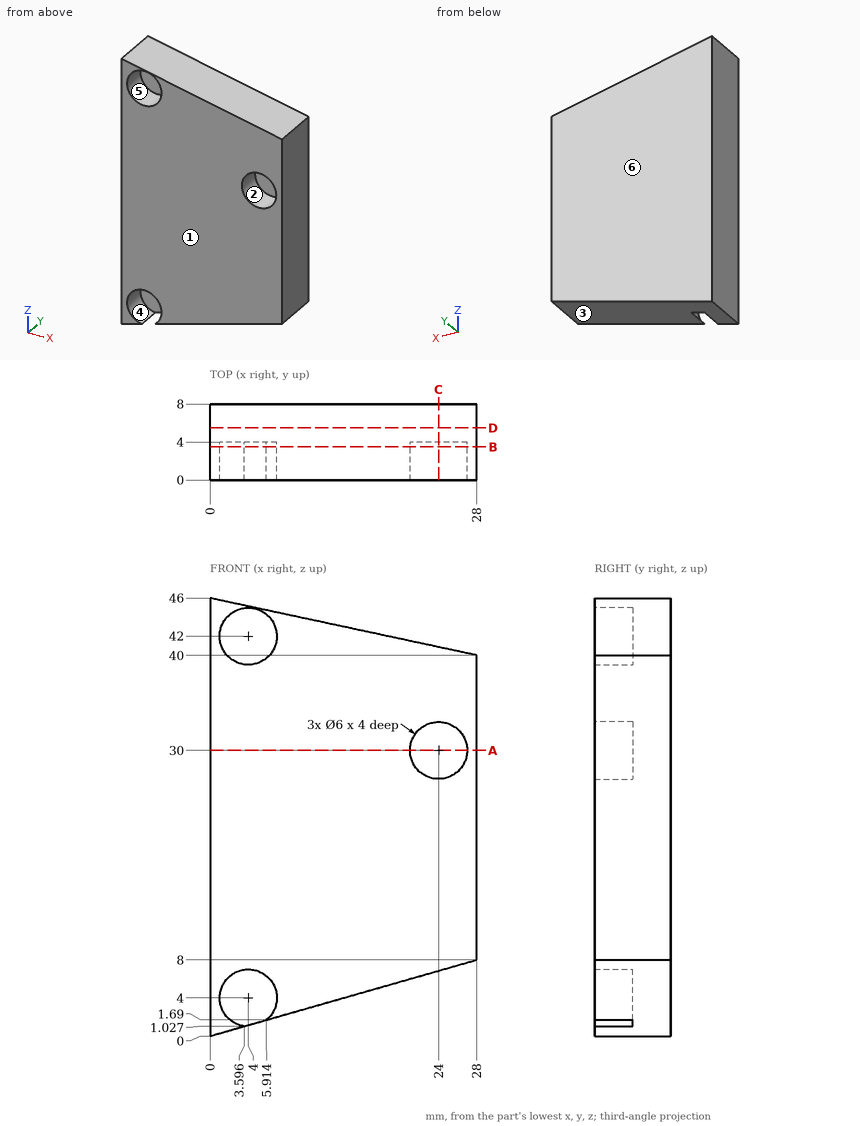
Source: three-view drawing plus pictorial views. Frame: mm from the lowest corner of the part. A direction names the side the tool comes from. Coordinates: 2 decimals unless noted, no trailing zeros. Loops run counter-clockwise (first coordinate to the right, second up) from the corner with the lowest first, then second, coordinate; pieces in that order, holes last. Notation, with made-up numbers: (53.25, 88) - (81.25, 88) arc R9 ccw to (81.25, 104) - close; hole circle Ø10 at (-4.75, 54.25). An arc over 180 degrees is marked (long way). One line per item, written item: value. Start each with the question number.
1. Section B-B (y = 3.5). Return the cut outline in (x, z) (1 decimal).
2. Section C-C (x = 24). Return the cut outline in (y, z).
3. Contact query for flat-ended pins moving along their axis: P1, Ø3.5, axis at x = 24, z = 30, coming from the -Y side; P2, Ø4, axis at x = 9.5, y = 1, coming from the -Z side. Output: stop coordinate, or through.
4. Section A-A (z = 30). Return the cut outline in (x, y).
5. Mould query, pull axis X, two halves, no side actions, for the marked faces 1, 2, 3 and 4. Classes: pulls with the +X half, pulls with the -X half, needs draft (parallel to the pull), parting line crosses it, or undercut.
6. Ray query, L1, parallel to X at y = 3.1, z = 30; L2, parallel to Y at x = 2, z = 6; L3, parallel to X at y = 3.5, z = 31. Return the intervals inside material, ascending.
7. Section D-D (y = 5.5). Return the cut outline in (x, z), and give its area (3 significant figures).
8. Set-up query: the marked faces 5 and 6. Return all of +Z, -Z, +X, -X, +Y, -Y with unobstructed straight access to the full face (end or side cutting, diameter ignored); none if empty.
Verdict:
1. outline: (0, 0) - (3.6, 1) arc R3 cw (long way) to (5.9, 1.7) - (28, 8) - (28, 40) - (0, 46) - close; hole circle Ø6 at (4, 42); hole circle Ø6 at (24, 30)
2. outline: (0, 6.86) - (8, 6.86) - (8, 40.86) - (0, 40.86) - (0, 33) - (4, 33) - (4, 27) - (0, 27) - close
3. P1: stops at y = 4
3. P2: stops at z = 2.14
4. outline: (0, 0) - (21, 0) - (21, 4) - (27, 4) - (27, 0) - (28, 0) - (28, 8) - (0, 8) - close
5. face 1: needs draft
5. face 2: undercut
5. face 3: pulls with the +X half
5. face 4: undercut
6. L1: x = 0 to 21, 27 to 28
6. L2: y = 4 to 8
6. L3: x = 0 to 21.17, 26.83 to 28
7. outline: (0, 0) - (28, 8) - (28, 40) - (0, 46) - close
7. area: 1,090 mm2
8. face 5: -Y
8. face 6: +Z, -Z, +X, -X, +Y
